CAD build for the part. Positions are in the model's coordinates, mm. Face numbers are marked on the shaded views. Give positions to 0.01 mm unless a question says otherwise; leave off trailing zeros. Answer in a Markdown table with one row per item. Add a question column.
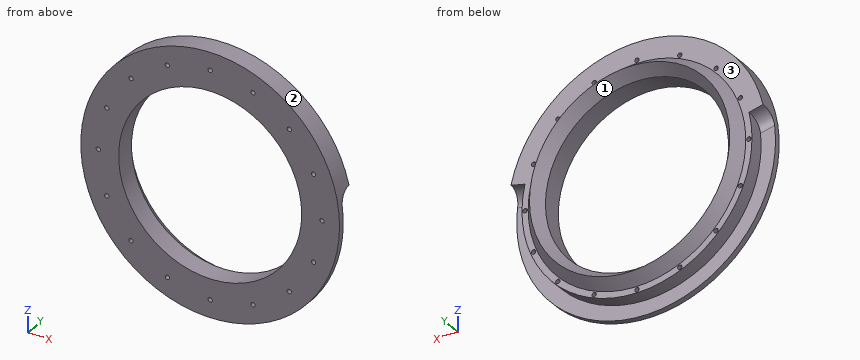
Solid Edge part; units mm, degrees
sketch "Sketch1" plane through (0, 0, 0) normal (0, -1, 0) x (1, 0, 0)
  circle A0 centre (0, 0) radius 40.4368
  circle A1 centre (0, 0) radius 50.8
extrude "Protrusion1" add sketch "Sketch1" along normal blind 8.89
sketch "Sketch2" plane through (0, 0, 0) normal (0, 0, 1) x (1, 0, 0)
  line L0 (44.2468, 5.08) -> (40.4368, 0)
  line L1 (40.4368, 0) -> (48.0568, 0)
  line L2 (44.2468, 5.08) -> (48.0568, 0)
revolve "RevolvedProtrusion1" add sketch "Sketch2" angle 360 about axis through (0, 0, 0) along (0, 1, 0)
sketch "Sketch3" plane through (0, 0, 0) normal (0, 1, 0) x (-1, 0, 0)
  circle A0 centre (0, 49.4284) radius 0.9525
extrude "Cutout1" cut sketch "Sketch3" against normal through all
pattern_circular "Pattern_2" count 16 over 360 about axis through (0, 0, 0) along (0, 1, 0) of "Cutout1"
sketch "Sketch4" plane through (0, 0, 0) normal (0, -1, 0) x (1, 0, 0)
  circle A0 centre (0, 0) radius 57.15
  circle A1 centre (0, 0) radius 50.8
extrude "Protrusion2" add sketch "Sketch4" along normal up to vertex (8.89 mm away)
sketch "Sketch5" plane through (0, 0, 0) normal (0, 1, 0) x (-1, 0, 0)
  line L0 (-55.6682, 12.9297) -> (-49.4828, 11.493)
  line L1 (55.6682, 12.9297) -> (49.4828, 11.493)
  arc A0 (49.4828, 11.493) -> (-49.4828, 11.493) centre (0, 0) cw
  arc A1 (55.6682, 12.9297) -> (-55.6682, 12.9297) centre (0, 0) cw
extrude "Cutout17" cut sketch "Sketch5" against normal blind 6.35
fillet "Round_2" radius 6.35 2 edges at (52.5755, -6.35, 12.2114) (-52.5755, -6.35, 12.2114)
Item 1: Mould opens along X. For the marked faces 1, 2 and 3 say: released by +X, released by -X, zero draft, split by the parting line, or undercut.
Item 2: Slice it at A-A, the plane y = -3. State how many separate pieces and enclosed holes the cut face has, then the cut area to 3 significant figures.
Item 3: Drop flat-ended pins along their axis: pin 1 Ø1.7 at (x, z) = (45.67, -18.92) entering from +Y; pin 2 Ø2.5 at (x, z) = (18.92, 45.67) entering from +Y; pin 3 Ø8 at (y, z) = (1.5, -10) entering from +X; pin 4 Ø4 at (y, z) = (-0.5, 6.5) entering from +X. Give the stop position or say it passes through.
Item 4: Probe L1, parallel to Z at x = -18.5, y = -7; L2, parallel to Y at x = 21, z = -48.5; L3, parallel to Z at x = 30, y = -4.5. List the from-to ranges inside material, lowest first. Write a range as from..to.
Answer key:
| question | item | result |
|---|---|---|
| 1 | face 1 | undercut |
| 1 | face 2 | split by the parting line |
| 1 | face 3 | zero draft |
| 2 | separate pieces | 1 |
| 2 | enclosed holes | 17 |
| 2 | area | 3,850 mm² |
| 3 | pin 1 | passes through |
| 3 | pin 2 | stops at y = 0 |
| 3 | pin 3 | stops at x = 50.41 |
| 3 | pin 4 | stops at x = 50.6 |
| 4 | L1 | z = -54.07..-46.52, -44.81..-35.96, 35.96..44.81, 46.52..54.07 |
| 4 | L2 | y = -8.89..-6.35 |
| 4 | L3 | z = -41..-27.11, 27.11..48.64 |
